Geometry check sheet. Reference: the model listing, model coordinates, mm. Face numbers are marked on the shaded views. Round coordinates to 2 decimals unless told otherwise and drop trailing zeros. Write each loop counter-clockwise with the first axis right and the second up, starting at its lowest first coordinate (ties: lowest second). Pieces come first, ordered by that corner, then holes.
Item 1: Scan lines: probe 1 along Y at (x, z) = (-14, 0); probe 2 along X at (y, z) = (21, 0); probe 3 along Y at (x, z) = (45, -4.5). Record each from-to range of solid material in increasing order.
Item 2: Depth check by flat-ended pin: P1, Ø6, axis at x = 40, z = 6.5, coming from the +Y side; P2, Ø5, axis at x = -0.5, z = 13.5, coming from the -Y side; P3, Ø6, axis at x = 12, y = 11, coming from the +Z side. Enter the tip coordinate at first touch or a pass-through.
Item 3: Cross-section at C-C (z = 6.5). State how many separate pieces and enclosed holes the cut face has, then the cut area to 3 significant figures.
Item 4: Cross-section at A-A (y = 42). Enter the section's corners in (x, z).
Item 5: Cross-section at B-B (x = 42.5). Enter the section's corners in (y, z).
Item 6: Draft check along Y on the marked faces 1, 2 and 3. Enter one of: pulls with the +Y half, pulls with the -Y half, needs draft (parallel to the pull), parting line crosses it, or undercut.
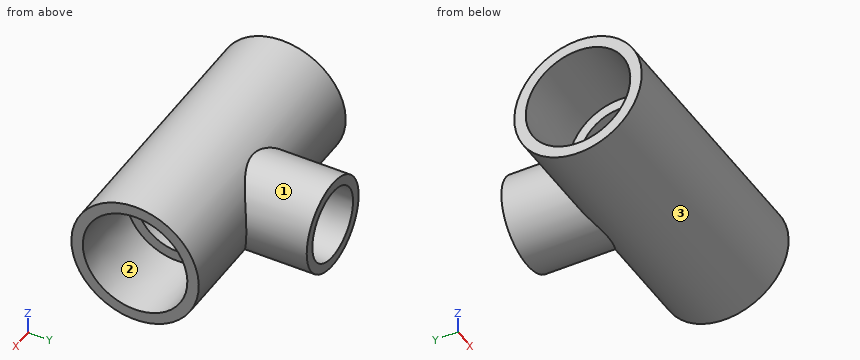
from build123d import *

# Parameters (mm, degrees)
SKETCH4_R           = 29.591
BOSS_EXTRUDE1_DEPTH = 51.308
SKETCH5_R           = 21.463
BOSS_EXTRUDE2_DEPTH = 25.908


with BuildPart() as part:
    # Sketch1 → Revolve1 (revolve)
    with BuildSketch(Plane.XY, mode=Mode.PRIVATE) as revolve1_sk:
        Polygon((-60.706, -29.591), (-25.654, -29.591), (-25.654, -24.0538), (-60.706, -24.2824), align=None)
        Polygon((60.706, -24.2824), (25.654, -24.0538), (25.654, -29.591), (60.706, -29.591), align=None)
    revolve(revolve1_sk.sketch.rotate(Axis((-60.706, 0, 0), (1, 0, 0)), 270), axis=Axis((-60.706, 0, 0), (1, 0, 0)))



with BuildPart() as body_2:
    # Sketch2 → Revolve2 (revolve)
    with BuildSketch(Plane.XY):
        Polygon((16.8275, 57.658), (16.637, 25.908), (21.463, 25.908), (21.463, 57.658), align=None)
    revolve(axis=Axis((0, 0, 0), (0, 1, 0)))


with BuildPart() as part_1:
    add(part.part)

    add(body_2.part)  # Boss-Extrude1 merges body 2
    # Sketch4 → Boss-Extrude1 (add)
    with BuildSketch(Plane(origin=(-25.654, 0, 0), x_dir=(0, 0, -1), z_dir=(1, 0, 0))):
        with Locations(Location((0, 0, 0), (0, 0, 180))):
            Circle(SKETCH4_R)
    extrude(amount=BOSS_EXTRUDE1_DEPTH)

    # Sketch5 → Boss-Extrude2 (add)
    with BuildSketch(Plane.XZ.offset(-25.908)):
        Circle(SKETCH5_R)
    extrude(amount=BOSS_EXTRUDE2_DEPTH)

    # Sketch6 → Cut-Revolve1 (revolve, cut)
    with BuildSketch(Plane.XY, mode=Mode.PRIVATE) as cut_revolve1_sk:
        Polygon((-60.706, -24.2824), (-25.654, -24.0538), (-25.654, -19.05), (25.654, -19.05), (25.654, -24.0538), (60.706, -24.2824), (60.706, 0), (-60.706, 0), align=None)
    revolve(cut_revolve1_sk.sketch.rotate(Axis((60.706, 0, 0), (-1, 0, 0)), 270), axis=Axis((60.706, 0, 0), (-1, 0, 0)), mode=Mode.SUBTRACT)

    # Sketch7 → Cut-Revolve2 (revolve, cut)
    with BuildSketch(Plane.XY):
        Polygon((16.8275, 57.658), (16.637, 25.908), (12.1539, 25.908), (12.1539, 0), (0, 0), (0, 57.658), align=None)
    revolve(axis=Axis((0, 0, 0), (0, 1, 0)), mode=Mode.SUBTRACT)


solid = part_1.part
Resolved:
1. probe 1: y = -29.59 to -19.05, 19.05 to 25.91
1. probe 2: x = -25.65 to -12.15, 12.15 to 25.65
1. probe 3: y = -29.25 to -23.76, 23.76 to 29.25
2. P1: stops at y = 29.38
2. P2: stops at y = -27.47
2. P3: stops at z = 28.49
3. separate pieces: 3
3. enclosed holes: 0
3. area: 1,940 mm2
4. outline: circle Ø42.93 at (0, 0); hole circle Ø33.47 at (0, 0)
5. outline: circle Ø59.18 at (0, 0); hole circle Ø48.33 at (0, 0)
6. face 1: needs draft
6. face 2: undercut
6. face 3: parting line crosses it
